Can you work these out from the model? Positions are in its coordinate system, mm. A direction names the side the tool comes from. Give positions to 0.01 mm unless a question says otherwise; leave off trailing zeros. Loops run counter-clockwise (first coordinate to the right, second up) from the corner with the lowest first, then second, coordinate; pieces in that order, holes last. Notation, with made-up numbers: M -1,-7 L 29,-7 A34 cw 29,30 Z; hole C -14,61 d4. An arc over 180 degrees is marked long. One line per item, written item: value. Start each with the question number.
Autodesk Inventor part; units mm, degrees
ref_plane "Work Plane1" through (0, 18, 0) normal (0, -1, 0) x (1, 0, 0)
ref_plane "YZ Plane" through (0, 0, 0) normal (1, 0, 0) x (0, 1, 0)
ref_plane "XZ Plane" through (0, 0, 0) normal (0, 1, 0) x (-1, 0, 0)
sketch "Sketch1" plane through (0, 0, 0) normal (0, 1, 0) x (-1, 0, 0)
  line L0 (-60, -124) -> (0, -124)
  line L1 (0, -124) -> (0, 0)
  line L2 (-58, -33) -> (-58, -122)
  line L3 (-58, -122) -> (-40, -122)
  line L4 (-40, -122) -> (-40, -124)
  line L5 (-2, -2) -> (-2, -122)
  line L6 (-2, -122) -> (-20, -122)
  line L7 (-20, -122) -> (-20, -124)
  line L8 (-60, -35) -> (-60, -124)
  line L9 (-30, -124) -> (-30, 0) construction
  line L10 (-60, -124) -> (-60, 0)
  line L11 (-58, -124) -> (-58, -2)
  line L12 (-2, -2) -> (-58, -2)
  line L13 (-60, 0) -> (0, 0)
  line L14 (-84, -5) -> (-84, -35)
  line L15 (-84, -35) -> (-58, -35)
  line L16 (-58, -35) -> (-58, 0)
  line L17 (-82, -7) -> (-82, -33)
  line L18 (-82, -33) -> (-58, -33)
  line L19 (-58, -33) -> (-58, -2)
  line L20 (-82, -7) -> (-60, -7)
  line L21 (-84, -5) -> (-60, -5)
  point P0 (-57.4156, -121.9986)
  point P1 (-58, -122)
  point P2 (-60, -35)
  point P3 (-58, -38)
  point P4 (-58, -33)
  point P5 (-60, -33)
  point P6 (-60, -35)
  point P7 (-58, -33)
  point P8 (-58, -35)
  point P9 (-58, -35)
  dimension "d0" = 60
  dimension "d5" = 2
  dimension "d6" = 20
  dimension "d38" = 2
  dimension "d39" = 60
  dimension "d46" = 2
  dimension "d47" = 2
  dimension "d48" = 2
  dimension "d50" = 30
  dimension "d51" = 2
  dimension "d64" = 2
  dimension "d66" = 26
extrude "Extrusion1" add sketch "Sketch1" against normal blind 2 contours L8 L15 L2 L11 L0 | L11 L3 L4 L0 | L10 L18 L2 L15 | L4 L3 L2 L11 L12 L5 L6 L7 L0 | L10 L13 L16 L11 L18 | L7 L6 L5 L12 L16 L13 L1 L0
extrude "Extrusion2" add sketch "Sketch1" along normal blind 40 contours L8 L15 L2 L11 L0 | L11 L3 L4 L0 | L10 L18 L2 L15 | L10 L13 L16 L11 L18 | L7 L6 L5 L12 L16 L13 L1 L0
sketch "Sketch2" plane through (0, -2, 0) normal (0, 0, 1) x (1, 0, 0)
  circle A0 centre (30, 17) radius 7
  line L0 (0, 42) -> (60, 42)
  line L1 (60, 0) -> (60, 42)
  point P0 (0, 2)
  point P1 (0, 42)
  point P2 (30, 42)
  dimension "d11" = 25
  dimension "d12" = 14
  dimension "d65" = 30
extrude "Extrusion3" cut sketch "Sketch2" against normal up to next
sketch "Sketch3" plane through (60, -2, 5.4121) normal (1, 0, 0) x (0, 0, -1)
  arc A0 (43.4121, 16) -> (61.4121, 16) centre (52.4121, 16) ccw
  line L0 (5.4121, 1.9762) -> (5.4121, 47)
  line L1 (61.4121, 16) -> (61.4121, 61)
  line L2 (61.4121, 61) -> (43.4121, 61)
  line L3 (43.4121, 61) -> (43.4121, 16)
  line L4 (5.4121, 47) -> (129.4107, 47) construction
  point P0 (5.4121, 2)
  point P1 (129.4107, 47)
  point P2 (5.4121, 0)
  dimension "d16" = 47
  dimension "d17" = 18
  dimension "d18" = 31
  dimension "d45" = 45
extrude "Extrusion4" cut sketch "Sketch3" against normal blind 2
ref_plane "Work Plane1" through (0, 18, 0) normal (0, -1, 0) x (1, 0, 0)
extrude "Extrusion7" add sketch "Sketch1" along normal up to surface (22 mm away) from surface at 18 contours L15 L14 L21 L10 L20 L17 L18
sketch "Sketch5" plane through (84, 18, -5) normal (1, 0, 0) x (0, 0, -1)
  line L0 (119, 22) -> (-5, 22)
  line L1 (33, 22) -> (33, -4)
  line L2 (-5, 22) -> (33, 22)
  line L3 (33, 22) -> (33, 19)
  line L4 (33, 19) -> (-5, 19)
  line L5 (-5, 19) -> (-5, 22)
  point P0 (-5, -18)
  dimension "d55" = 3
extrude "Extrusion8" cut sketch "Sketch5" against normal up to surface (26 mm away)
sketch "Sketch6" plane through (60, 18, -5) normal (0, 0, 1) x (1, 0, 0)
  circle A0 centre (14, 4) radius 1.75
  line L0 (24, 0) -> (24, 19)
  line L1 (0, 0) -> (24, 0)
  point P0 (-60, -18)
  dimension "d58" = 3.5
  dimension "d59" = 10
  dimension "d60" = 4
extrude "Extrusion9" cut sketch "Sketch6" against normal blind 10
fillet "Fillet1" radius 2 5 edges at (30, -2, 0) (0, 19, 0) (60, 17.5, 0) (84, 27.5, -35) (84, 27.5, -5)
sketch "Sketch7" plane through (0, 0, -122) normal (-1, 0, 0) x (0, 0, 1)
  line L0 (120, -2) -> (0, -2)
  line L1 (23, -2) -> (23, 23.6999)
  arc A0 (23, 23.6999) -> (30.364, 28.0218) centre (23, 32.1346) ccw
  arc A1 (67.8122, 50) -> (30.364, 28.0218) centre (67.8122, 7.1072) ccw
  line L2 (-2, 40) -> (120, 40)
  line L3 (-2, 50) -> (-2, 0)
  line L4 (67.8122, 50) -> (-2, 50)
  line L5 (-2, 50) -> (-2, -2)
  line L6 (-2, -2) -> (23, -2)
  point P0 (122, 0)
  point P1 (0, 50)
  point P2 (120, 40)
  point P3 (40.283, 40)
  point P4 (67.8122, 50)
  dimension "d67" = 25
extrude "Extrusion10" cut sketch "Sketch7" against normal through all
sketch "Sketch8" plane through (0, 0, -99) normal (0, 0, -1) x (-1, 0, 0)
  line L0 (0, 23.6999) -> (0, -2)
  line L1 (0, -2) -> (-12.5, -2)
  line L2 (-12.5, -2) -> (-12.5, 23.6999)
  line L3 (-12.5, 23.6999) -> (0, 23.6999)
  line L4 (0, 23.6999) -> (0, -2)
  line L5 (-60, -2) -> (-60, 23.6999)
  line L6 (-60, -2) -> (-47.5, -2)
  line L7 (-47.5, -2) -> (-47.5, 24.1231)
  line L8 (-47.5, 24.1231) -> (-60, 24.1231)
  line L9 (-60, 24.1231) -> (-60, -2)
  point P0 (0, 0)
  point P1 (-60, 23.6999)
  dimension "d70" = 35
extrude "Extrusion11" add sketch "Sketch8" along normal blind 2
properties part number "tension_sensor_cover" material "ABS Plastic"
Q1. If we section it at B-B, the plane x = 74: Write out the boundary of the cut face in (y, z).
Q2. I need wall thicknesses on line 1 along X through (y, z) = (21, -58.5); line 2 along X through (y, z) = (33, -30); line 3 along Z through (x, y) = (4.5, 10). Which ranges of each line are inside material? Lowest first, please.
Q3. If we section it at C-C, the plane x = 30: Write out the boundary of the cut face in (y, z), plus the area to 3 significant figures.
Q4. If we section it at D-D, the plane y = 12.5: Write out the boundary of the cut face in (x, z), plus the area to 3 significant figures.
Q5. If we mould it in two halves opening along Z, with no side actions, what happens to faces 5 (the face through (52, 12, -99)), 6 (the face through (75.669, 22.526, -5.986)), 7 (the face through (6, 11, -101))? For each: released by +Z, released by -Z, zero draft, split by the parting line, or undercut.
Q6. For P1, Ø12, axis at x = 32, z = -59, coming from the +Y side; P2, Ø5, axis at y = 2.5, z = -38, coming from the +X side; P3, Ø2, axis at x = 74, y = 22, coming from the -Z side, each with a flat end and sliding along its axis, tell me the tip position at first contact or that it passes through.
Q7. Which directions (+Z, -Z, +X, -X, +Y, -Y) give clear straight access to the entire face, cutting with the end or side of a thin tool? Please do faces 1 (the face through (7, 12, -99)), 2 (the face through (58.99, 24.83, -94.78)), 3 (the face through (71, 27, -5)), 4 (the face through (59.5, 37, -19.1)).
Q8. If we section it at A-A, the plane z = -20.5: Write out the boundary of the cut face in (x, y).
Response:
1. outline: M 18,-35 L 37,-35 L 37,-33 L 18,-33 Z; M 18,-7 L 20.25,-7 L 20.25,-5 L 18,-5 Z; M 23.75,-7 L 37,-7 L 37,-5 L 23.75,-5 Z
2. line 1: 0 to 2, 58 to 60
2. line 2: 0 to 2, 58 to 60, 82 to 84
2. line 3: -101 to -99, -2 to 0
3. outline: M -2,-99 L 0,-99 L 0,-2 L 8,-2 L 8,0 L 0,0 A2 ccw -2,-2 Z; M 22,-2 L 40,-2 L 40,0 L 22,0 Z
3. area: 249 mm^2
4. outline: M 0,-101 L 12.5,-101 L 12.5,-99 L 2,-99 L 2,-2 L 23.46,-2 L 23.46,0 L 2,0 A2 ccw 0,-2 Z; M 36.54,-2 L 58,-2 L 58,-38.13 L 60,-38.13 L 60,-2 A2 ccw 58,0 L 36.54,0 Z; M 47.5,-101 L 60,-101 L 60,-55.87 L 58,-55.87 L 58,-99 L 47.5,-99 Z
4. area: 495 mm^2
5. face 5: undercut
5. face 6: zero draft
5. face 7: released by -Z
6. P1: y = 0
6. P2: x = 60
6. P3: z = -35
7. face 1: +Y
7. face 2: +X, -X, +Y
7. face 3: +Z, +X, +Y, -Y
7. face 4: +Z, +X, +Y
8. outline: M 0,-2 L 60,-2 L 60,37 L 58,37 L 58,0 L 2,0 L 2,40 L 0,40 Z; M 82,18 L 84,18 L 84,37 L 82,37 Z
